CAD build for the part. Positions are in the model's coordinates, mm. A direction names the side the tool comes from. Round coordinates to 2 decimals unless told otherwise and drop trailing zeros. Order: outer loops, then holes, each group sorted by start corner. A loop starts at its lowest first (then second) coordinate and runs counter-clockwise, first axis right, second up. Notation, with made-up numbers: (83, 35.25) - (109, 35.25) arc R20 cw to (109, 55.25) - close; hole circle Ø3 at (-23.75, 13.5). An arc over 180 degrees is marked (long way). Write item = value, one per line.
from build123d import *

# Parameters (mm, degrees)
BOSS_EXTRUDE1_DEPTH = 57.15
SKETCH2_R           = 2.0193
CUT_EXTRUDE1_DEPTH  = 19.05
SKETCH4_R           = 7.057360916
SKETCH4_R_2         = 5.125
CUT_EXTRUDE2_DEPTH  = 7.112


with BuildPart() as part:
    # Sketch1 → Boss-Extrude1 (new, symmetric)
    with BuildSketch(Plane.XY):
        Polygon((4.7625, 2.749630657), (0, 5.499261314), (-4.7625, 2.749630657), (-4.7625, -2.749630657), (0, -5.499261314), (4.7625, -2.749630657), align=None)
    extrude(amount=BOSS_EXTRUDE1_DEPTH, both=True)

    # Sketch2 → Cut-Extrude1 (cut)
    with BuildSketch(Plane(origin=(0, 0, -57.15), x_dir=(-1, 0, 0), z_dir=(0, 0, -1))):
        Circle(SKETCH2_R)
    cut_extrude1 = extrude(amount=-CUT_EXTRUDE1_DEPTH, mode=Mode.SUBTRACT)

    # Mirror1: Cut-Extrude1 across plane
    add(cut_extrude1.mirror(Plane.XY), mode=Mode.SUBTRACT)

    # Sketch4 → Cut-Extrude2 (cut)
    with BuildSketch(Plane.XY.offset(57.15)):
        Circle(SKETCH4_R)
        Circle(SKETCH4_R_2, mode=Mode.SUBTRACT)
    cut_extrude2 = extrude(amount=-CUT_EXTRUDE2_DEPTH, mode=Mode.SUBTRACT)

    # Mirror2: Cut-Extrude2 across plane
    add(cut_extrude2.mirror(Plane.XY), mode=Mode.SUBTRACT)


solid = part.part
(1) Band-saw the part on A-A on y = 0. List the corners of the cut face in (x, z), plus the area to 3 significant figures.
Solved:
outline = (-4.76, -57.15) - (-2.02, -57.15) - (-2.02, -38.1) - (2.02, -38.1) - (2.02, -57.15) - (4.76, -57.15) - (4.76, 57.15) - (2.02, 57.15) - (2.02, 38.1) - (-2.02, 38.1) - (-2.02, 57.15) - (-4.76, 57.15) - close
area = 935 mm²
(2) Pull direction Y, two halves, no side cores. Call faces 1 (the flat face through (4.762, 0, 1)), 2 (the flat face through (0, 0, -38.1)), 3 (the cylindrical face through (-1.926, 0.607, 47.758)), 4 (the flat face through (2.348, -4.144, 0.8)): released by +Y, released by -Y, zero draft, split by the parting line, or undercut.
Solved:
face_1 = zero draft
face_2 = undercut
face_3 = undercut
face_4 = released by -Y
(3) Probe line 1 along Y through (x, z) = (0, 50.75) (3 decimals); line 2 along Y through (x, z) = (0, 44); line 3 along Y through (x, z) = (1.25, 19.5). List the from-to ranges inside material, lowest first.
Solved:
line_1 = -5.125 to -2.019, 2.019 to 5.125
line_2 = -5.5 to -2.02, 2.02 to 5.5
line_3 = -4.78 to 4.78
(4) Tool access for faces 5 (the flat face through (-2.2, 0.1, -57.15)), 6 (the flat face through (0, 0, 38.1)), 7 (the cylindrical face through (-1.926, 0.607, -47.758)): list every direction of +Z, -Z, +X, -X, +Y, -Y with a clear straight run to the whole face (end or side of a thin tool).
Solved:
face_5 = -Z, +X, -X, +Y, -Y
face_6 = +Z
face_7 = -Z
(5) Band-saw the part on B-B on z = -22. List the corners of the cut face in (x, y), plus the area to 3 significant figures.
Solved:
outline = (-4.76, -2.75) - (0, -5.5) - (4.76, -2.75) - (4.76, 2.75) - (0, 5.5) - (-4.76, 2.75) - close
area = 78.6 mm²
(6) Drop flat-ended pins along their axis: pin 1 (1.2 mm diameter, centred on x = 0.5, y = 1, fed in from +Z); pin 2 (0.5 mm diameter, centred on x = 0, y = -5.5, fed in from +Z); pin 3 (1.5 mm diameter, centred on x = 1.5, z = 38, fed in from -Y). Give the stop position or say it passes through.
Solved:
pin_1 = 38.1
pin_2 = 50.04
pin_3 = -5.07
